The model under review builds one solid part; all positions refer to its coordinate system, in mm. Give positions to 0.01 mm unless a question says otherwise; leave off trailing zeros. Loops run counter-clockwise (first coordinate to the right, second up) from the corner with the lowest first, then second, coordinate; pieces in that order, holes last. Notation, with made-up numbers: (-0.5, -24) -> (22.5, -24) arc R25 ccw to (22.5, 0) -> close; hole circle Ø11 at (71, -12.5). An arc over 180 degrees is marked (long way). Write each question's results on one line, items separated by ' | '. Start each with the question number.
Q1. We need section D-D (y = 0.7). Write out the cut boundary in (x, z).
Q2. We need section B-B (z = 0). Write out the cut boundary in (x, y), plus the area to 3 significant figures.
Q3. Insertion check: pin 1 Ø3 at (x, z) = (-0.5, -1) entering from -Y. The pin has a flat end and moves straight along its axis. Give the tip position at first contact, or say it passes through.
Q4. Wall thickness on L1, parallel to X at y = 2.15, z = 0; L2, parallel to X at y = 0.75, z = 0: over which ranges is each line inside the solid? List them lowest first. Write a range as [from, to].
Q5. Mouldability with a two-part tool opening along Z and no side actions: class faces 1 (the face through (1.95, 0.82, -0.61)), 2 (the face through (0.245, 1.465, 1.103)), 3 (the face through (-2, 1.524, -1)) as released by +Z, released by -Z, zero draft, split by the parting line, or undercut.
Q6. We need section C-C (y = 2.45). Write out the cut boundary in (x, z).
Q7. We need section A-A (x = 0). Write out the cut boundary in (y, z).
from build123d import *

# Parameters (mm, degrees)
SKETCH1_R             = 2.0447
BOSS_EXTRUDE1_DEPTH   = 1.524
SKETCH2_R             = 2.7813
BOSS_EXTRUDE2_DEPTH   = 1.5748
F_4_40_TAPPED_HOLE1_D = 2.2606
CHAMFER1_SIZE         = 0.127


with BuildPart() as part:
    # Sketch1 → Boss-Extrude1 (new body)
    with BuildSketch(Plane(origin=(0, 0, 0), x_dir=(1, 0, 0), z_dir=(0, 1, 0))):
        Circle(SKETCH1_R)
    extrude(amount=BOSS_EXTRUDE1_DEPTH)

    # Sketch2 → Boss-Extrude2 (add)
    with BuildSketch(Plane(origin=(0, 1.524, 0), x_dir=(1, 0, 0), z_dir=(0, 1, 0))):
        Circle(SKETCH2_R)
    extrude(amount=BOSS_EXTRUDE2_DEPTH)

    # #4-40 Tapped Hole1 (through all)
    with Locations(Plane(origin=(0, 3.0988, 0), x_dir=(1, 0, 0), z_dir=(0, 1, 0))):
        with Locations((0, 0)):
            Hole(F_4_40_TAPPED_HOLE1_D / 2)

    # Chamfer1
    chamfer1_edges = [part.edges().sort_by_distance(p)[0] for p in [
        (1.1303, 3.0988, 0),
        (-2.0447, 0, 0),
        (-2.7813, 3.0988, 0),
    ]]
    chamfer(chamfer1_edges, length=CHAMFER1_SIZE)


solid = part.part
Output:
1) outline: circle Ø4.09 at (0, 0); hole circle Ø2.26 at (0, 0)
2) outline: (-2.78, 1.52) -> (-2.04, 1.52) -> (-2.04, 0.13) -> (-1.92, 0) -> (-1.13, 0) -> (-1.13, 2.97) -> (-1.26, 3.1) -> (-2.65, 3.1) -> (-2.78, 2.97) -> close; (1.13, 0) -> (1.92, 0) -> (2.04, 0.13) -> (2.04, 1.52) -> (2.78, 1.52) -> (2.78, 2.97) -> (2.65, 3.1) -> (1.26, 3.1) -> (1.13, 2.97) -> close | area: 7.94 mm2
3) pin 1: y = 0
4) L1: [-2.78, -1.13], [1.13, 2.78] | L2: [-2.04, -1.13], [1.13, 2.04]
5) face 1: split by the parting line | face 2: undercut | face 3: zero draft
6) outline: circle Ø5.56 at (0, 0); hole circle Ø2.26 at (0, 0)
7) outline: (0, -1.92) -> (0.13, -2.04) -> (1.52, -2.04) -> (1.52, -2.78) -> (2.97, -2.78) -> (3.1, -2.65) -> (3.1, -1.26) -> (2.97, -1.13) -> (0, -1.13) -> close; (0, 1.13) -> (2.97, 1.13) -> (3.1, 1.26) -> (3.1, 2.65) -> (2.97, 2.78) -> (1.52, 2.78) -> (1.52, 2.04) -> (0.13, 2.04) -> (0, 1.92) -> close
